from build123d import *

# Parameters (mm, degrees)
SKETCH1_R           = 22.5
BOSS_EXTRUDE1_DEPTH = 3


with BuildPart() as part:
    # Sketch1 → Boss-Extrude1 (new body)
    with BuildSketch(Plane(origin=(0, 0, 0), x_dir=(1, 0, 0), z_dir=(0, 1, 0))):
        with Locations(Location((0, 0, 0), (0, 0, 270))):
            Circle(SKETCH1_R)
        with BuildLine():
            ThreePointArc((12.858274793, 13.988022353), (7.926678354, 17.267535154), (2.224901963, 18.869282214))
            add(Edge.make_bspline(
                [(11.875562109, 3.901413152), (12.889627473, 3.505325226), (11.613923706, 10.788790468), (5.151799162, 17.696017864), (2.224901963, 18.869282214)],
                knots=[0, 0, 0, 0, 0.363857402, 1, 1, 1, 1], degree=3))
            add(Edge.make_bspline(
                [(0.778823269, 3.412247693), (5.685303017, 7.967969249), (11.875562109, 3.901413152)],
                knots=[0, 0, 0, 1, 1, 1], degree=2))
            ThreePointArc((0.778823269, 3.412247693), (1.339392013, 3.233578364), (1.862112268, 2.963534697))
            add(Edge.make_bspline(
                [(1.862112268, 2.963534697), (7.080742295, 3.142252132), (10.068013486, 1.06766484), (11.854735792, -3.964245112)],
                knots=[0, 0, 0, 0, 1, 1, 1, 1], degree=3))
            add(Edge.make_bspline(
                [(11.854735792, -3.964245112), (15.892673154, 4.806059129), (12.858274793, 13.988022353)],
                knots=[0, 0, 0, 1, 1, 1], degree=2))
        make_face(mode=Mode.SUBTRACT)
        with BuildLine():
            ThreePointArc((0.778823269, -3.412247693), (1.339392013, -3.233578364), (1.862112268, -2.963534697))
            add(Edge.make_bspline(
                [(1.862112268, -2.963534697), (1.614088771, -9.654321405), (-5.638574802, -11.156006194)],
                knots=[0, 0, 0, 1, 1, 1], degree=2))
            add(Edge.make_bspline(
                [(-5.638574802, -11.156006194), (-6.635703756, -11.592982231), (-0.583457308, -15.84111111), (8.870102109, -16.155846354), (11.769354144, -14.915840675)],
                knots=[0, 0, 0, 0, 0.363857402, 1, 1, 1, 1], degree=3))
            ThreePointArc((11.769354144, -14.915840675), (6.604983185, -17.814999218), (0.79885216, -18.983198762))
            add(Edge.make_bspline(
                [(-11.185708668, -5.579419467), (-7.839419958, -14.63621396), (0.79885216, -18.983198762)],
                knots=[0, 0, 0, 1, 1, 1], degree=2))
            add(Edge.make_bspline(
                [(0.778823269, -3.412247693), (-2.784933102, -7.228748683), (-6.36420756, -7.874113658), (-11.185708668, -5.579419467)],
                knots=[0, 0, 0, 0, 1, 1, 1, 1], degree=3))
        make_face(mode=Mode.SUBTRACT)
        with BuildLine():
            ThreePointArc((-0.79885216, 18.983198762), (-6.604983185, 17.814999218), (-11.769354144, 14.915840675))
            add(Edge.make_bspline(
                [(5.638574802, 11.156006194), (6.635703756, 11.592982231), (0.583457308, 15.84111111), (-8.870102109, 16.155846354), (-11.769354144, 14.915840675)],
                knots=[0, 0, 0, 0, 0.363857402, 1, 1, 1, 1], degree=3))
            add(Edge.make_bspline(
                [(-1.862112268, 2.963534697), (-1.614088771, 9.654321405), (5.638574802, 11.156006194)],
                knots=[0, 0, 0, 1, 1, 1], degree=2))
            ThreePointArc((-1.862112268, 2.963534697), (-1.339392013, 3.233578364), (-0.778823269, 3.412247693))
            add(Edge.make_bspline(
                [(-0.778823269, 3.412247693), (2.784933102, 7.228748683), (6.36420756, 7.874113658), (11.185708668, 5.579419467)],
                knots=[0, 0, 0, 0, 1, 1, 1, 1], degree=3))
            add(Edge.make_bspline(
                [(11.185708668, 5.579419467), (7.839419958, 14.63621396), (-0.79885216, 18.983198762)],
                knots=[0, 0, 0, 1, 1, 1], degree=2))
        make_face(mode=Mode.SUBTRACT)
        with BuildLine():
            ThreePointArc((-13.988022353, 12.858274793), (-17.267535154, 7.926678354), (-18.869282214, 2.224901963))
            add(Edge.make_bspline(
                [(-3.901413152, 11.875562109), (-3.505325226, 12.889627473), (-10.788790468, 11.613923706), (-17.696017864, 5.151799162), (-18.869282214, 2.224901963)],
                knots=[0, 0, 0, 0, 0.363857402, 1, 1, 1, 1], degree=3))
            add(Edge.make_bspline(
                [(-3.412247693, 0.778823269), (-7.967969249, 5.685303017), (-3.901413152, 11.875562109)],
                knots=[0, 0, 0, 1, 1, 1], degree=2))
            ThreePointArc((-3.412247693, 0.778823269), (-3.233578364, 1.339392013), (-2.963534697, 1.862112268))
            add(Edge.make_bspline(
                [(-2.963534697, 1.862112268), (-3.142252132, 7.080742295), (-1.06766484, 10.068013486), (3.964245112, 11.854735792)],
                knots=[0, 0, 0, 0, 1, 1, 1, 1], degree=3))
            add(Edge.make_bspline(
                [(3.964245112, 11.854735792), (-4.806059129, 15.892673154), (-13.988022353, 12.858274793)],
                knots=[0, 0, 0, 1, 1, 1], degree=2))
        make_face(mode=Mode.SUBTRACT)
        with BuildLine():
            ThreePointArc((-18.983198762, -0.79885216), (-17.814999218, -6.604983185), (-14.915840675, -11.769354144))
            add(Edge.make_bspline(
                [(-11.156006194, 5.638574802), (-11.592982231, 6.635703756), (-15.84111111, 0.583457308), (-16.155846354, -8.870102109), (-14.915840675, -11.769354144)],
                knots=[0, 0, 0, 0, 0.363857402, 1, 1, 1, 1], degree=3))
            add(Edge.make_bspline(
                [(-2.963534697, -1.862112268), (-9.654321405, -1.614088771), (-11.156006194, 5.638574802)],
                knots=[0, 0, 0, 1, 1, 1], degree=2))
            ThreePointArc((-2.963534697, -1.862112268), (-3.233578364, -1.339392013), (-3.412247693, -0.778823269))
            add(Edge.make_bspline(
                [(-3.412247693, -0.778823269), (-7.228748683, 2.784933102), (-7.874113658, 6.36420756), (-5.579419467, 11.185708668)],
                knots=[0, 0, 0, 0, 1, 1, 1, 1], degree=3))
            add(Edge.make_bspline(
                [(-5.579419467, 11.185708668), (-14.63621396, 7.839419958), (-18.983198762, -0.79885216)],
                knots=[0, 0, 0, 1, 1, 1], degree=2))
        make_face(mode=Mode.SUBTRACT)
        with BuildLine():
            ThreePointArc((-12.858274793, -13.988022353), (-7.926678354, -17.267535154), (-2.224901963, -18.869282214))
            add(Edge.make_bspline(
                [(-11.875562109, -3.901413152), (-12.889627473, -3.505325226), (-11.613923706, -10.788790468), (-5.151799162, -17.696017864), (-2.224901963, -18.869282214)],
                knots=[0, 0, 0, 0, 0.363857402, 1, 1, 1, 1], degree=3))
            add(Edge.make_bspline(
                [(-0.778823269, -3.412247693), (-5.685303017, -7.967969249), (-11.875562109, -3.901413152)],
                knots=[0, 0, 0, 1, 1, 1], degree=2))
            ThreePointArc((-0.778823269, -3.412247693), (-1.339392013, -3.233578364), (-1.862112268, -2.963534697))
            add(Edge.make_bspline(
                [(-1.862112268, -2.963534697), (-7.080742295, -3.142252132), (-10.068013486, -1.06766484), (-11.854735792, 3.964245112)],
                knots=[0, 0, 0, 0, 1, 1, 1, 1], degree=3))
            add(Edge.make_bspline(
                [(-11.854735792, 3.964245112), (-15.892673154, -4.806059129), (-12.858274793, -13.988022353)],
                knots=[0, 0, 0, 1, 1, 1], degree=2))
        make_face(mode=Mode.SUBTRACT)
        with BuildLine():
            ThreePointArc((13.988022353, -12.858274793), (17.267535154, -7.926678354), (18.869282214, -2.224901963))
            add(Edge.make_bspline(
                [(3.901413152, -11.875562109), (3.505325226, -12.889627473), (10.788790468, -11.613923706), (17.696017864, -5.151799162), (18.869282214, -2.224901963)],
                knots=[0, 0, 0, 0, 0.363857402, 1, 1, 1, 1], degree=3))
            add(Edge.make_bspline(
                [(3.412247693, -0.778823269), (7.967969249, -5.685303017), (3.901413152, -11.875562109)],
                knots=[0, 0, 0, 1, 1, 1], degree=2))
            ThreePointArc((3.412247693, -0.778823269), (3.233578364, -1.339392013), (2.963534697, -1.862112268))
            add(Edge.make_bspline(
                [(2.963534697, -1.862112268), (3.142252132, -7.080742295), (1.06766484, -10.068013486), (-3.964245112, -11.854735792)],
                knots=[0, 0, 0, 0, 1, 1, 1, 1], degree=3))
            add(Edge.make_bspline(
                [(-3.964245112, -11.854735792), (4.806059129, -15.892673154), (13.988022353, -12.858274793)],
                knots=[0, 0, 0, 1, 1, 1], degree=2))
        make_face(mode=Mode.SUBTRACT)
        with BuildLine():
            ThreePointArc((3.412247693, 0.778823269), (3.233578364, 1.339392013), (2.963534697, 1.862112268))
            add(Edge.make_bspline(
                [(2.963534697, 1.862112268), (9.654321405, 1.614088771), (11.156006194, -5.638574802)],
                knots=[0, 0, 0, 1, 1, 1], degree=2))
            add(Edge.make_bspline(
                [(11.156006194, -5.638574802), (11.592982231, -6.635703756), (15.84111111, -0.583457308), (16.155846354, 8.870102109), (14.915840675, 11.769354144)],
                knots=[0, 0, 0, 0, 0.363857402, 1, 1, 1, 1], degree=3))
            ThreePointArc((14.915840675, 11.769354144), (17.814999218, 6.604983185), (18.983198762, 0.79885216))
            add(Edge.make_bspline(
                [(5.579419467, -11.185708668), (14.63621396, -7.839419958), (18.983198762, 0.79885216)],
                knots=[0, 0, 0, 1, 1, 1], degree=2))
            add(Edge.make_bspline(
                [(3.412247693, 0.778823269), (7.228748683, -2.784933102), (7.874113658, -6.36420756), (5.579419467, -11.185708668)],
                knots=[0, 0, 0, 0, 1, 1, 1, 1], degree=3))
        make_face(mode=Mode.SUBTRACT)
    extrude(amount=BOSS_EXTRUDE1_DEPTH)


solid = part.part
Source: CAD feature listing. Evaluate the final solid. Frame: model axes, mm. Round coordinates to 2 decimals unless told otherwise and drop trailing zeros. Write item = value, one per line. Start each with the question number.
(1) Ray query, line 1 along Z through (x, y) = (-16, 1.8); line 2 along X through (y, z) = (0.5, -16.5); line 3 along Z through (x, y) = (-17.5, 2.45) (3 decimals). Return the intervals inside material, ascending. Write a range as from..to.
(2) Section query A-A, the plane x = -10. State how many separate pieces and enclosed holes the cut face has, plus the area to 3 significant figures.
(3) Pull-direction query (Z, two-part tool) for faces 1 (the face through (0, 0, 0)), 2 (the face through (3.237, 1.479, 1.332)), 3 (the face through (-8.618, 1.479, 20.784)); classes: +Z half, -Z half, draft (parallel to the pull), parting line (faces both ways), or undercut.
(4) Pin query (flat end, axial travel): pin 1 (1 mm diameter, centred on y = 2, z = -2, fed in from +X); pin 2 (1.5 mm diameter, centred on y = 2.5, z = -17.5, fed in from +X). Return the tip coordinate at first contact, or that it passes through.
Conclusion:
q1.line_1 = -15.82..-10.25, -6.21..-3.85, 10.25..15.82
q1.line_2 = -15.3..-9.42, 3.21..5.69, 9.42..15.3
q1.line_3 = -14.142..-7.399, -4.505..-1.786, 7.399..14.142
q2.separate_pieces = 7
q2.enclosed_holes = 0
q2.area = 51.4 mm2
q3.face_1 = draft
q3.face_2 = undercut
q3.face_3 = parting line
q4.pin_1 = 22.45
q4.pin_2 = 15.02
